Build history of the part. All positions in model axes, mm. A direction names the side the tool comes from. Coordinates: 2 decimals unless noted, no trailing zeros. Loops run counter-clockwise (first coordinate to the right, second up) from the corner with the lowest first, then second, coordinate; pieces in that order, holes last.
(1) Slice it at B-B (y = -7.5). Give the cut face in (x, z) (3 decimals).
(2) Wall check: L1, parallel to Y at x = 15.5, z = 1.8; L2, parallel to X at y = -13, z = -27.5; L3, parallel to Y at x = 24.5, z = -33. Give the ranges that are in metal, low to high.
(3) Slice it at D-D (y = 15.5). Give the cut face in (x, z), and give its area (3 significant figures).
(4) Flat gauge pins, fed straight in: P1, Ø1.8, axis at x = -15.5, y = -15.5, coming from the +Z side; P2, Ø1.3, axis at x = 27.5, y = 10.5, coming from the +Z side; P3, Ø12, axis at x = -8, y = -17, coming from the -Z side; P4, Ø10, axis at x = 27, z = -27, coming from the +Y side. Where does each tip first touch, or does it go through?
(5) Slice it at C-C (z = -27.5). Give the cut face in (x, y), and give its area (3 significant figures).
(6) Two-plate mould, pull along Y, no slides. Class faces 6 (the face through (-31, 9.35, -26)), 7 (the face through (29, 10, -40)), 8 (the face through (12.5, 0, 1)), 9 (the face through (29, -6.35, -26)): pulls with the +Y half, pulls with the -Y half, needs draft (parallel to the pull), parting line crosses it, or undercut.
(7) Tool access for faces 1 (the face through (24, -16.35, -29)), 2 (the face through (31, 9.35, -26)), 3 (the face through (-27, -11, -25)), 4 (the face through (-12.5, 0, 1)), 5 (the face through (-29, -6.35, -26)): list every direction of +Z, -Z, +X, -X, +Y, -Y with a clear straight run to the whole face (end or side of a thin tool).
(8) Slice it at A-A (x = -33.5). Give the cut face in (y, z) (3 decimals).
from build123d import *

# Parameters (mm, degrees)
SKETCH1_W                   = 52
SKETCH1_H                   = 52
SKETCH1_W_2                 = 42
SKETCH1_H_2                 = 42
BOSS_EXTRUDE1_DEPTH         = 8
SKETCH3_W                   = 5
SKETCH3_H                   = 10
BOSS_EXTRUDE3_DEPTH         = 32
SKETCH4_W                   = 15
SKETCH4_H                   = 3
BOSS_EXTRUDE4_DEPTH         = 15
MIRROR2_COPY_1_SKETCH_W     = 15
MIRROR2_COPY_1_SKETCH_H     = 3
MIRROR2_COPY_1_DEPTH        = 15
SKETCH2_W                   = 52
SKETCH2_H                   = 52
SKETCH2_W_2                 = 25
SKETCH2_H_2                 = 25
BOSS_EXTRUDE2_DEPTH         = 3
F_1_4_0_25_DIAMETER_HOLE1_D = 6.35
RIB1_REACH                  = 84.25
SKETCH9_WALL_W              = 180.146400996
SKETCH9_WALL_H              = 5
MIRROR5_COPY_1_REACH        = 84.25
MIRROR5_COPY_1_SKETCH_W     = 180.146400996
MIRROR5_COPY_1_SKETCH_H     = 5
F_3_0MM_DOWEL_HOLE1_D       = 3
BOSS_EXTRUDE5_DEPTH         = 1.5
BOSS_EXTRUDE6_START         = -15
BOSS_EXTRUDE6_DEPTH         = 1.5
MIRROR7_COPY_1_DEPTH        = 1.5
MIRROR7_START               = -15
MIRROR7_COPY_2_DEPTH        = 1.5
RIB12_REACH                 = 67.784
SKETCH13_WALL_W             = 156.23938331
SKETCH13_WALL_H             = 3
MIRROR9_COPY_1_REACH        = 67.784
MIRROR9_COPY_1_SKETCH_W     = 156.23938331
MIRROR9_COPY_1_SKETCH_H     = 3


with BuildPart() as part:
    # Sketch1 → Boss-Extrude1 (new body)
    with BuildSketch(Plane.XY):
        Rectangle(SKETCH1_W, SKETCH1_H)
        Rectangle(SKETCH1_W_2, SKETCH1_H_2, mode=Mode.SUBTRACT)
    extrude(amount=-BOSS_EXTRUDE1_DEPTH)

    # Sketch3 → Boss-Extrude3 (add)
    with BuildSketch(Plane(origin=(0, 0, -8), x_dir=(-1, 0, 0), z_dir=(0, 0, -1))):
        with Locations((-23.5, 11.35)):
            Rectangle(SKETCH3_W, SKETCH3_H)
        with Locations((-23.5, -11.35)):
            Rectangle(SKETCH3_W, SKETCH3_H)
    boss_extrude3 = extrude(amount=BOSS_EXTRUDE3_DEPTH)

    # Sketch4 → Boss-Extrude4 (add)
    with BuildSketch(Plane(origin=(26, 0, 0), x_dir=(0, 0, -1), z_dir=(1, 0, 0))):
        with Locations((32.5, -7.85)):
            Rectangle(SKETCH4_W, SKETCH4_H)
    boss_extrude4 = extrude(amount=BOSS_EXTRUDE4_DEPTH)

    # Mirror1: Boss-Extrude4 across plane
    add(boss_extrude4.mirror(Plane.ZX))

    # Mirror2: Boss-Extrude3, Boss-Extrude4 across plane
    add(boss_extrude3.mirror(Plane(origin=(0, 0, 0), x_dir=(0, 0, 1), z_dir=(1, 0, 0))))
    add(boss_extrude4.mirror(Plane(origin=(0, 0, 0), x_dir=(0, 0, 1), z_dir=(1, 0, 0))))

    # Mirror2 copy 1 sketch → Mirror2 copy 1 (add)
    with BuildSketch(Plane(origin=(-26, 0, 0), x_dir=(0, 0, -1), z_dir=(-1, 0, 0))):
        with Locations((32.5, -7.85)):
            Rectangle(MIRROR2_COPY_1_SKETCH_W, MIRROR2_COPY_1_SKETCH_H)
    extrude(amount=MIRROR2_COPY_1_DEPTH)

    # Sketch2 → Boss-Extrude2 (add)
    with BuildSketch(Plane.XY):
        Rectangle(SKETCH2_W, SKETCH2_H)
        Rectangle(SKETCH2_W_2, SKETCH2_H_2, mode=Mode.SUBTRACT)
    extrude(amount=BOSS_EXTRUDE2_DEPTH)

    # 1/4 (0.25) Diameter Hole1 (through all)
    with Locations(Plane(origin=(0, -9.35, 0), x_dir=(-1, 0, 0), z_dir=(0, -1, 0))):
        with Locations((33.5, 32.5)):
            f_1_4_0_25_diameter_hole1 = Hole(F_1_4_0_25_DIAMETER_HOLE1_D / 2)

    # Mirror3: 1/4 (0.25) Diameter Hole1 across plane
    add(f_1_4_0_25_diameter_hole1.mirror(Plane(origin=(0, 0, 0), x_dir=(0, 0, 1), z_dir=(1, 0, 0))), mode=Mode.SUBTRACT)

    # Sketch9 wall → Rib1 (add, up to next)
    with BuildSketch(Plane(origin=(-26, -21.175, -12.825), x_dir=(0, 0.707106781187, -0.707106781187), z_dir=(0, -0.707106781187, -0.707106781187)), mode=Mode.PRIVATE) as rib1_sk1:
        with Locations((0, 2.5)):
            Rectangle(SKETCH9_WALL_W, SKETCH9_WALL_H)
    rib1_tool1 = extrude(rib1_sk1.sketch, amount=-RIB1_REACH, mode=Mode.PRIVATE) - part.part
    rib1 = rib1_tool1.solids().sort_by_distance((-26, -21.175, -12.825))[0]
    add(rib1)

    # Mirror4: Rib1 across plane
    add(rib1.mirror(Plane.ZX))

    # Mirror5: Rib1 across plane
    add(rib1.mirror(Plane(origin=(0, 0, 0), x_dir=(0, 0, 1), z_dir=(1, 0, 0))))

    # Mirror5 copy 1 sketch → Mirror5 copy 1 (add, up to next)
    with BuildSketch(Plane(origin=(26, 21.175, -12.825), x_dir=(0, -0.707106781187, -0.707106781187), z_dir=(0, 0.707106781187, -0.707106781187)), mode=Mode.PRIVATE) as mirror5_copy_1_sk1:
        with Locations((0, 2.5)):
            Rectangle(MIRROR5_COPY_1_SKETCH_W, MIRROR5_COPY_1_SKETCH_H)
    mirror5_copy_1_tool1 = extrude(mirror5_copy_1_sk1.sketch, amount=-MIRROR5_COPY_1_REACH, mode=Mode.PRIVATE) - part.part
    add(mirror5_copy_1_tool1.solids().sort_by_distance((26, 21.175, -12.825))[0])

    # Ø3.0mm Dowel Hole1 (through all)
    with Locations(Plane(origin=(0, 0, 0), x_dir=(-1, 0, 0), z_dir=(0, 0, -1))):
        with Locations((15.5, -15.5), (-15.5, -15.5), (-15.5, 15.5), (15.5, 15.5)):
            Hole(F_3_0MM_DOWEL_HOLE1_D / 2)

    # Sketch12 → Boss-Extrude5 (add)
    with BuildSketch(Plane.XY.offset(-25)):
        Polygon((-30.5, -9.35), (-26, -13.85), (-26, -9.35), align=None)
    boss_extrude5 = extrude(amount=-BOSS_EXTRUDE5_DEPTH)

    # Sketch12<3> → Boss-Extrude6 (add)
    with BuildSketch(Plane.XY.offset(-25).offset(BOSS_EXTRUDE6_START)):
        Polygon((-30.5, -9.35), (-26, -13.85), (-26, -9.35), align=None)
    boss_extrude6 = extrude(amount=BOSS_EXTRUDE6_DEPTH)

    # Mirror6: Boss-Extrude5, Boss-Extrude6 across plane
    add(boss_extrude5.mirror(Plane(origin=(0, 0, 0), x_dir=(0, 0, 1), z_dir=(1, 0, 0))))
    add(boss_extrude6.mirror(Plane(origin=(0, 0, 0), x_dir=(0, 0, 1), z_dir=(1, 0, 0))))

    # Mirror7: Boss-Extrude5, Boss-Extrude6 across plane
    add(boss_extrude5.mirror(Plane.ZX))
    add(boss_extrude6.mirror(Plane.ZX))

    # Mirror7 copy 1 sketch → Mirror7 copy 1 (add)
    with BuildSketch(Plane(origin=(0, 0, -25), x_dir=(-1, 0, 0), z_dir=(0, 0, 1))):
        Polygon((-30.5, -9.35), (-26, -13.85), (-26, -9.35), align=None)
    extrude(amount=-MIRROR7_COPY_1_DEPTH)

    # Mirror7 copy 2 sketch → Mirror7 copy 2 (add)
    with BuildSketch(Plane(origin=(0, 0, -25), x_dir=(-1, 0, 0), z_dir=(0, 0, 1)).offset(MIRROR7_START)):
        Polygon((-30.5, -9.35), (-26, -13.85), (-26, -9.35), align=None)
    extrude(amount=MIRROR7_COPY_2_DEPTH)

    # Sketch13 wall → Rib12 (add, up to next)
    with BuildSketch(Plane(origin=(-33.5, -6.35, -16.5), x_dir=(-0.661621637087, 0, -0.749837855365), z_dir=(-0.749837855365, 0, 0.661621637087)), mode=Mode.PRIVATE) as rib12_sk1:
        with Locations((0, 1.5)):
            Rectangle(SKETCH13_WALL_W, SKETCH13_WALL_H)
    rib12_tool1 = extrude(rib12_sk1.sketch, amount=-RIB12_REACH, mode=Mode.PRIVATE) - part.part
    rib12 = rib12_tool1.solids().sort_by_distance((-33.5, -6.35, -16.5))[0]
    add(rib12)

    # Mirror8: Rib12 across plane
    add(rib12.mirror(Plane.ZX))

    # Mirror9: Rib12 across plane
    add(rib12.mirror(Plane(origin=(0, 0, 0), x_dir=(0, 0, 1), z_dir=(1, 0, 0))))

    # Mirror9 copy 1 sketch → Mirror9 copy 1 (add, up to next)
    with BuildSketch(Plane(origin=(33.5, 6.35, -16.5), x_dir=(0.661621637087, 0, -0.749837855365), z_dir=(0.749837855365, 0, 0.661621637087)), mode=Mode.PRIVATE) as mirror9_copy_1_sk1:
        with Locations((0, 1.5)):
            Rectangle(MIRROR9_COPY_1_SKETCH_W, MIRROR9_COPY_1_SKETCH_H)
    mirror9_copy_1_tool1 = extrude(mirror9_copy_1_sk1.sketch, amount=-MIRROR9_COPY_1_REACH, mode=Mode.PRIVATE) - part.part
    add(mirror9_copy_1_tool1.solids().sort_by_distance((33.5, 6.35, -16.5))[0])


solid = part.part
Response values:
1. outline: (-41, -40) - (-21, -40) - (-21, 0) - (-12.5, 0) - (-12.5, 3) - (-26, 3) - (-26, -8) - (-41, -25) - close; (12.5, 0) - (21, 0) - (21, -40) - (41, -40) - (41, -25) - (26, -8) - (26, 3) - (12.5, 3) - close; hole circle Ø6.35 at (-33.5, -32.5); hole circle Ø6.35 at (33.5, -32.5)
2. L1: y = -26 to -17, -14 to 14, 17 to 26
2. L2: x = -26 to -21, 21 to 26
2. L3: y = -16.35 to -6.35, 6.35 to 16.35
3. outline: (-26, -40) - (-21, -40) - (-21, 0) - (-17, 0) - (-17, 3) - (-26, 3) - close; (-14, 0) - (14, 0) - (14, 3) - (-14, 3) - close; (17, 0) - (21, 0) - (21, -40) - (26, -40) - (26, 3) - (17, 3) - close
3. area: 538 mm2
4. P1: passes through
4. P2: stops at z = -25
4. P3: stops at z = -8
4. P4: stops at y = 16.35
5. outline: (-41, -9.35) - (-26, -9.35) - (-26, -16.35) - (-21, -16.35) - (-21, -6.35) - (-41, -6.35) - close; (-41, 6.35) - (-21, 6.35) - (-21, 16.35) - (-26, 16.35) - (-26, 9.35) - (-41, 9.35) - close; (21, -16.35) - (26, -16.35) - (26, -9.35) - (41, -9.35) - (41, -6.35) - (21, -6.35) - close; (21, 6.35) - (41, 6.35) - (41, 9.35) - (26, 9.35) - (26, 16.35) - (21, 16.35) - close
5. area: 380 mm2
6. face 6: pulls with the +Y half
6. face 7: needs draft
6. face 8: undercut
6. face 9: undercut
7. face 1: -Z, +X, -X, -Y
7. face 2: +X, +Y
7. face 3: +Z, -X, -Y
7. face 4: +Z, -Z
7. face 5: -Z, +X, -X
8. outline: (-9.35, -40) - (-6.35, -40) - (-6.35, -35.675) - (-9.35, -35.675) - close; (-9.35, -29.325) - (-6.35, -29.325) - (-6.35, -16.5) - (-9.35, -16.5) - close; (6.35, -40) - (9.35, -40) - (9.35, -35.675) - (6.35, -35.675) - close; (6.35, -29.325) - (9.35, -29.325) - (9.35, -16.5) - (6.35, -16.5) - close
